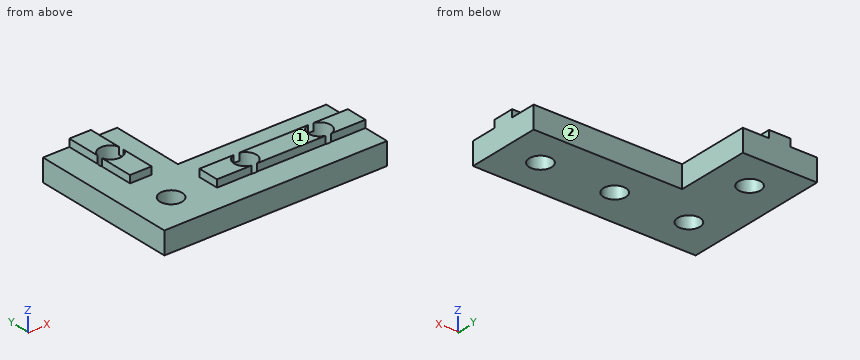
from build123d import *

# Parameters (mm, degrees)
BOSS_EXTRU_1_DEPTH      = 3
ESQUISSE2_W             = 2.9
ESQUISSE2_H             = 10
ESQUISSE2_W_2           = 20
ESQUISSE2_H_2           = 2.9
BOSS_EXTRU_2_DEPTH      = 1
ESQUISSE3_R             = 1.5
ENL_V_MAT_EXTRU_1_DEPTH = 5


with BuildPart() as part:
    # Esquisse1 → Boss.-Extru.1 (new body)
    with BuildSketch(Plane.XY):
        Polygon((0, 0), (30, 0), (30, 10), (10, 10), (10, 20), (0, 20), align=None)
    extrude(amount=BOSS_EXTRU_1_DEPTH)

    # Esquisse2 → Boss.-Extru.2 (add)
    with BuildSketch(Plane.XY.offset(3)):
        with Locations((5, 15)):
            Rectangle(ESQUISSE2_W, ESQUISSE2_H)
        with Locations((20, 5)):
            Rectangle(ESQUISSE2_W_2, ESQUISSE2_H_2)
    extrude(amount=BOSS_EXTRU_2_DEPTH)

    # Esquisse3 → Enlèv. mat.-Extru.1 (cut, through all)
    with BuildSketch(Plane(origin=(0, 0, 0), x_dir=(-1, 0, 0), z_dir=(0, 0, -1))):
        with Locations((-25, 5)):
            Circle(ESQUISSE3_R)
        with Locations((-15, 5)):
            Circle(ESQUISSE3_R)
        with Locations((-5, 15)):
            Circle(ESQUISSE3_R)
        with Locations((-5, 5)):
            Circle(ESQUISSE3_R)
    extrude(amount=-ENL_V_MAT_EXTRU_1_DEPTH, mode=Mode.SUBTRACT)


solid = part.part
Input: part model. Units: mm. Frame: model coordinates. Face numbers are marked on the shaded views. A direction names the side the tool comes from. Give positions to 0.01 mm unless a question says otherwise; leave off trailing zeros. Order: outer loops, then holes, each group sorted by start corner. A loop starts at its lowest first (then second) coordinate and runs counter-clockwise, first axis right, second up. Notation, with made-up numbers: M 21,-25.5 L 60,-25.5 A20 cw 60,9.5 Z; hole C 79,19.5 d3. An arc over 180 degrees is marked long. Answer as a JSON object with one key per item and string values.
1. First-contact query: P1, Ø1.5, axis at x = 21, y = 4, coming from the -Z side; P2, Ø1.1, axis at x = 18.5, z = 3.5, coming from the +Y side; P3, Ø0.5, axis at y = 12, z = 3.5, coming from the +X side; P4, Ø2, axis at y = 15.5, z = 1.5, coming from the +X side. Flat tips, straight axial feed; report the tip coordinate or a pass-through.
Result sheet:
{"P1": "z = 0", "P2": "y = 10", "P3": "x = 6.45", "P4": "x = 10"}
2. Cut plane B-B, the plane x = 5. Output: boundary loops of the cut face in (y, z).
Result sheet:
{"outline": "M 0,0 L 3.5,0 L 3.5,3 L 0,3 Z; M 6.5,0 L 13.5,0 L 13.5,4 L 10,4 L 10,3 L 6.5,3 Z; M 16.5,0 L 20,0 L 20,4 L 16.5,4 Z"}
3. Cut plane D-D, the plane z = 0.5. Output: boundary loops of the cut face in (x, y).
Result sheet:
{"outline": "M 0,0 L 30,0 L 30,10 L 10,10 L 10,20 L 0,20 Z; hole C 5,5 d3; hole C 5,15 d3; hole C 15,5 d3; hole C 25,5 d3"}
4. Reachability of the marked faces 1 and 2 from +Z, -Z, +X, -X, +Y, -Y: full face, straight path, thin tool, end or side. Return the list, or none.
Result sheet:
{"face 1": "+Z, +X, -X, +Y, -Y", "face 2": "+Z, -Z, +X, +Y"}
5. Cut plane A-A, the plane x = 15. Output: boundary loops of the cut face in (y, z).
Result sheet:
{"outline": "M 0,0 L 3.5,0 L 3.5,3 L 0,3 Z; M 6.5,0 L 10,0 L 10,3 L 6.5,3 Z"}
6. Ray query, line 1 (Y direction, x = 5, z = 0.8); line 2 (X direction, y = 5, z = 3.05); line 3 (Y direction, x = 25, z = 1.3). Return the intervals inside material, ascending. Write a range as [from, to].
Result sheet:
{"line 1": "[0, 3.5], [6.5, 13.5], [16.5, 20]", "line 2": "[10, 13.5], [16.5, 23.5], [26.5, 30]", "line 3": "[0, 3.5], [6.5, 10]"}
